Verification items for the finished model (mm, model axes). A direction names the side the tool comes from. Round coordinates to 2 decimals unless told otherwise and drop trailing zeros. Order: outer loops, then holes, each group sorted by start corner. A loop starts at its lowest first (then second) coordinate and runs counter-clockwise, first axis right, second up. Notation, with made-up numbers: M -18.5,-36 L 3.5,-36 A22 ccw 3.5,-25 Z; hole C 28.25,31 d11. An arc over 180 degrees is marked long. Use CSV: the item, a comma, the result in double quotes. Start each with the question number.
Q1. Sectioned sample at B-B (y = 0). Enter the section's corners in (x, z), and give its area (3 significant figures).
Q2. Gauge pin test, flat ends, axial feed: pin 1 Ø1.1 at (x, z) = (1, 26) entering from -Y; pin 2 Ø10 at (y, z) = (-11.5, 34.5) entering from -X; pin 3 Ø12 at (y, z) = (11.5, 23) entering from -X. Record the tip position at first contact, or that the pin passes through.
Q3. Sectioned sample at C-C (x = 0). Enter the section's corners in (y, z), and give its area (3 significant figures).
Q4. Sectioned sample at A-A (z = 14). Enter the section's corners in (x, y), and give its area (3 significant figures).
Q5. Mould release check, pull along Y, two halves, no side actions. Record for faces 5 (the face through (-9.43, -16.12, 22.32)), 6 (the face through (18.673, -0.11, 22.325)), 7 (the face through (-14.92, -8.64, 22.68)), 8 (the face through (8, -8, 35)): +Y half, -Y half, draft (parallel to the pull), parting line (faces both ways), or undercut.
Q6. Set-up check for faces 1 (the face through (-16.454, -7.299, 22.675)), 2 (the face through (0, 17.24, 23)), 3 (the face through (14.55, -10.6, 22.68)), 4 (the face through (9.936, 3.129, 37.465)): record each of +Z, -Z, +X, -X, +Y, -Y from which the full face is reachable in a straight line by a thin tool's end or side.
Q7. Sectioned sample at D-D (y = -13). Enter the section's corners in (x, z), and give its area (3 significant figures).
Q8. Scan lines: line 1 (Z direction, x = 7.5, y = -7.5); line 2 (Z direction, x = -10, y = 15.5); line 3 (Y direction, x = -2, z = 32). Record each from-to range of solid material in increasing order.
```python
from build123d import *

# Parameters (mm, degrees)
CROQUIS1_R              = 20
SALIENTE_EXTRUIR5_DEPTH = 5
CROQUIS6_R              = 16.544256432
SALIENTE_EXTRUIR6_DEPTH = 5
CROQUIS7_R              = 18.673739687
SALIENTE_EXTRUIR7_DEPTH = 25
CROQUIS8_W              = 3.810951086
CROQUIS8_H              = 2.867445731
CORTAR_EXTRUIR2_DEPTH   = 25
CROQUIS9_R              = 10.417374192
SALIENTE_EXTRUIR9_DEPTH = 5


with BuildPart() as part:
    # Croquis1 → Saliente-Extruir5 (new body)
    with BuildSketch(Plane.XY):
        Circle(CROQUIS1_R)
    extrude(amount=SALIENTE_EXTRUIR5_DEPTH)

    # Croquis6 → Saliente-Extruir6 (add)
    with BuildSketch(Plane.XY.offset(5)):
        Circle(CROQUIS6_R)
    extrude(amount=SALIENTE_EXTRUIR6_DEPTH)

    # Croquis7 → Saliente-Extruir7 (add)
    with BuildSketch(Plane.XY.offset(10)):
        Circle(CROQUIS7_R)
    extrude(amount=SALIENTE_EXTRUIR7_DEPTH)

    # Croquis8 → Cortar-Extruir2 (cut)
    with BuildSketch(Plane.XY.offset(35)):
        with Locations((0, 18.673739686)):
            Rectangle(CROQUIS8_W, CROQUIS8_H)
        Polygon((16.460835604, 11.703921503), (13.977554757, 10.270198637), (15.8830303, 6.969818184), (18.366311148, 8.403541049), align=None)
        Polygon((18.366311148, -8.403541049), (15.8830303, -6.969818184), (13.977554757, -10.270198637), (16.460835604, -11.703921503), align=None)
        with Locations((0, -18.673739686)):
            Rectangle(CROQUIS8_W, CROQUIS8_H)
        Polygon((-16.460835604, -11.703921503), (-13.977554757, -10.270198637), (-15.8830303, -6.969818184), (-18.366311148, -8.403541049), align=None)
        Polygon((-18.366311148, 8.403541049), (-15.8830303, 6.969818184), (-13.977554757, 10.270198637), (-16.460835604, 11.703921503), align=None)
    extrude(amount=-CORTAR_EXTRUIR2_DEPTH, mode=Mode.SUBTRACT)

    # Croquis9 → Saliente-Extruir9 (add)
    with BuildSketch(Plane.XY.offset(35)):
        Circle(CROQUIS9_R)
    extrude(amount=SALIENTE_EXTRUIR9_DEPTH)


solid = part.part
```
Verdict:
1,outline,"M -20,0 L 20,0 L 20,5 L 16.54,5 L 16.54,10 L 18.67,10 L 18.67,35 L 10.42,35 L 10.42,40 L -10.42,40 L -10.42,35 L -18.67,35 L -18.67,10 L -16.54,10 L -16.54,5 L -20,5 Z"
1,area,"1,400 mm²"
2,pin 1,"stops at y = -17.24"
2,pin 2,"stops at x = -17.51"
2,pin 3,"stops at x = -17.85"
3,outline,"M -20,0 L 20,0 L 20,5 L 16.54,5 L 16.54,10 L 17.24,10 L 17.24,35 L 10.42,35 L 10.42,40 L -10.42,40 L -10.42,35 L -17.24,35 L -17.24,10 L -16.54,10 L -16.54,5 L -20,5 Z"
3,area,"1,330 mm²"
4,outline,"M -17.04,-7.64 L -15.88,-6.97 L -13.98,-10.27 L -15.13,-10.94 A18.67 ccw -1.91,-18.58 L -1.91,-17.24 L 1.91,-17.24 L 1.91,-18.58 A18.67 ccw 15.13,-10.94 L 13.98,-10.27 L 15.88,-6.97 L 17.04,-7.64 A18.67 ccw 17.04,7.64 L 15.88,6.97 L 13.98,10.27 L 15.13,10.94 A18.67 ccw 1.91,18.58 L 1.91,17.24 L -1.91,17.24 L -1.91,18.58 A18.67 ccw -15.13,10.94 L -13.98,10.27 L -15.88,6.97 L -17.04,7.64 A18.67 ccw Z"
4,area,"1,060 mm²"
5,face 5,"-Y half"
5,face 6,"parting line"
5,face 7,"undercut"
5,face 8,"draft"
6,face 1,"+Z, -Y"
6,face 2,"+Z, +Y"
6,face 3,"+Z, +X"
6,face 4,"+Z"
7,outline,"M -15.2,0 L 15.2,0 L 15.2,5 L 10.23,5 L 10.23,10 L 13.41,10 L 13.41,35 L -13.41,35 L -13.41,10 L -10.23,10 L -10.23,5 L -15.2,5 Z"
7,area,"925 mm²"
8,line 1,"z = 0 to 35"
8,line 2,"z = 0 to 5, 10 to 35"
8,line 3,"y = -18.57 to 18.57"
